from build123d import *

# Parameters (mm, degrees)
SKETCH1_R           = 7.5
SKETCH1_W           = 6.85
SKETCH1_H           = 6.85
BOSS_EXTRUDE1_DEPTH = 6
SKETCH2_R           = 11
SKETCH2_R_2         = 7.5
BOSS_EXTRUDE2_DEPTH = 1
BOSS_EXTRUDE3_START = 6
SKETCH1_2_R         = 7.5
SKETCH1_2_W         = 6.85
SKETCH1_2_H         = 6.85
BOSS_EXTRUDE3_DEPTH = 2


with BuildPart() as part:
    # Sketch1 → Boss-Extrude1 (new, symmetric)
    with BuildSketch(Plane.XY):
        Circle(SKETCH1_R)
        Rectangle(SKETCH1_W, SKETCH1_H, mode=Mode.SUBTRACT)
    extrude(amount=BOSS_EXTRUDE1_DEPTH, both=True)

    # Sketch2 → Boss-Extrude2 (add)
    with BuildSketch(Plane(origin=(0, 0, -6), x_dir=(-1, 0, 0), z_dir=(0, 0, -1))):
        Circle(SKETCH2_R)
        Circle(SKETCH2_R_2, mode=Mode.SUBTRACT)
    extrude(amount=-BOSS_EXTRUDE2_DEPTH)

    # Sketch1<2> → Boss-Extrude3 (add)
    with BuildSketch(Plane.XY.offset(BOSS_EXTRUDE3_START)):
        with Locations(Location((0, 0, 0), (0, 0, 180))):
            Circle(SKETCH1_2_R)
        Rectangle(SKETCH1_2_W, SKETCH1_2_H, mode=Mode.SUBTRACT)
        Rectangle(SKETCH1_2_W, SKETCH1_2_H)
    extrude(amount=BOSS_EXTRUDE3_DEPTH)


solid = part.part
Input: part model. Units: mm. Frame: model coordinates. A direction names the side the tool comes from. Give positions to 0.01 mm unless a question says otherwise; leave off trailing zeros. Write each loop counter-clockwise with the first axis right and the second up, starting at its lowest first coordinate (ties: lowest second). Pieces come first, ordered by that corner, then holes.
Q1. Section D-D, the plane x = -6. Output: boundary loops of the cut face in (y, z), plus the area to 3 significant figures.
Q2. Pull-direction query (X, two-part tool) for faces 3 (the face through (0, 3.425, 0)), 4 (the face through (2.38, -10.74, -5.51)), 5 (the face through (-7.2, 2.6, -5)), 6 (the face through (0, -3.425, 0)); classes: pulls with the +X half, pulls with the -X half, needs draft (parallel to the pull), parting line crosses it, or undercut.
Q3. First-contact query: P1, Ø3.5, axis at y = -0.5, z = -0.5, coming from the -X side; P2, Ø1.5, axis at x = -3, z = -4.5, coming from the +Y side; P3, Ø5.5, axis at x = -0.5, y = 0, coming from the -Z side. Flat tips, straight axial feed; report the tip coordinate or a pass-through.
Q4. Set-up query: faces 1 (the face through (0, 0, 6)), 2 (the face through (0, 0, 8)). Return all of +Z, -Z, +X, -X, +Y, -Y with unobstructed straight access to the full face (end or side cutting, diameter ignored); none if empty.
Q5. Material intervals for probe 1 along X at (y, z) = (-0.25, -1.75) (3 decimals); probe 2 along X at (y, z) = (-4.5, 7); probe 3 along Z at (x, y) = (7, -3.5), sorted ascending.
Q6. Section A-A, the plane y = 0. Output: boundary loops of the cut face in (x, z) (3 decimals), plus the area to 3 significant figures.
Q7. Section B-B, the plane z = 5.5. Output: boundary loops of the cut face in (x, y) (3 decimals).
Filled in:
1. outline: (-9.22, -6) - (9.22, -6) - (9.22, -5) - (4.5, -5) - (4.5, 8) - (-4.5, 8) - (-4.5, -5) - (-9.22, -5) - close
1. area: 135 mm2
2. face 3: undercut
2. face 4: parting line crosses it
2. face 5: needs draft
2. face 6: undercut
3. P1: stops at x = -7.5
3. P2: stops at y = 10.73
3. P3: stops at z = 6
4. face 1: -Z
4. face 2: +Z, +X, -X, +Y, -Y
5. probe 1: x = -7.496 to -3.425, 3.425 to 7.496
5. probe 2: x = -6 to 6
5. probe 3: z = -6 to -5
6. outline: (-11, -6) - (-3.425, -6) - (-3.425, 6) - (3.425, 6) - (3.425, -6) - (11, -6) - (11, -5) - (7.5, -5) - (7.5, 8) - (-7.5, 8) - (-7.5, -5) - (-11, -5) - close
6. area: 135 mm2
7. outline: circle Ø15 at (0, 0); hole (-3.425, -3.425) - (3.425, -3.425) - (3.425, 3.425) - (-3.425, 3.425) - close
